Work out the finished part from the listing and answer in its coordinate system (mm). A direction names the side the tool comes from. Give positions to 0.01 mm unless a question says otherwise; leave off trailing zeros. Loops run counter-clockwise (first coordinate to the right, second up) from the corner with the lowest first, then second, coordinate; pieces in that order, holes last. Notation, with made-up numbers: (8, -21) - (58, -21) arc R16 cw to (58, -4) - close; hole circle Ø10 at (62, 6). An arc over 180 degrees is marked (long way). One line per question, with ' | ' between items. Start each with the question number.
1. Each of these flat-tipped pins is pushed along its axis until it touches: pin 1 (1 mm diameter, centred on y = 274, z = 6.5, fed in from -X); pin 2 (1 mm diameter, centred on y = 146, z = 16.5, fed in from -X); pin 3 (3 mm diameter, centred on x = -100.5, z = 47.5, fed in from +Y). Where does it stop, or does it pass through?
2. Which of the six approach directions +Z, -Z, +X, -X, +Y, -Y give full straight-line access (tool end or side, diameter ignored) to faces 1 (the face through (-55, 8, 78.536)), 2 (the face through (-128.253, 304.011, 9.435))?
3. Section D-D (x = -122) is taken. Determine the outline of the cut face in (y, z), plus the area to 3 significant figures.
4. Section C-C (y = 94) is taken. Determine the outline of the cut face in (x, z).
5. Section A-A (z = 29.5) is taken. Determine the outline of the cut face in (x, y).
6. Section B-B (x = -60.5) is taken. Determine the outline of the cut face in (y, z), plus the area to 3 significant figures.
7. Find the intervals of material crossed by line 1 (Z direction, x = 52.85, y = 8); line 2 (Y direction, x = 21, z = 52); line 3 (Z direction, x = -121, y = 312), in increasing order.
Autodesk Inventor part; units mm, degrees
ref_plane "YZ Plane" through (0, 0, 0) normal (1, 0, 0) x (0, 1, 0)
ref_plane "XZ Plane" through (0, 0, 0) normal (0, 1, 0) x (-1, 0, 0)
ref_plane "XY Plane" through (0, 0, 0) normal (0, 0, 1) x (1, 0, 0)
sketch "Sketch1" plane through (0, 0, 0) normal (0, 1, 0) x (-1, 0, 0)
  line L0 (159.7591, 78.536) -> (-52.9659, 78.536)
  line L1 (-52.9659, 78.536) -> (-52.9659, -60.184)
  line L2 (-52.9659, -60.184) -> (159.7591, -60.184)
  line L3 (159.7591, -60.184) -> (159.7591, 78.536)
  point P0 (0, 0)
  dimension "d0" = 138.72
  dimension "d1" = 212.725
extrude "Extrusion1" add sketch "Sketch1" along normal blind 16
sketch "Sketch2" plane through (0, 16, 0) normal (0, 1, 0) x (1, 0, 0)
  line L0 (-159.7591, -78.536) -> (52.9659, -78.536)
  line L1 (52.9659, -78.536) -> (52.9659, 60.184)
  line L2 (52.9659, 60.184) -> (-159.7591, 60.184)
  line L3 (-159.7591, 60.184) -> (-159.7591, -78.536)
  line L4 (-159.7591, 60.184) -> (-159.7591, -78.536)
  line L5 (-159.7591, -9.176) -> (52.9659, -9.176)
  line L6 (52.9659, -78.536) -> (52.9659, 60.184)
  circle A0 centre (-122.3691, -9.176) radius 5.89
  line L7 (-122.3691, -9.176) -> (-128.2591, -9.176)
  point P0 (0, 0)
  dimension "d4" = 11.78
  dimension "d5" = 31.5
extrude "Extrusion2" add sketch "Sketch2" along normal blind 584.2 contours A0 L5 | L5 A0
sketch "Sketch3" plane through (52.9659, 0, 78.536) normal (1, 0, 0) x (0, 0, -1)
  line L0 (0, 0) -> (138.72, 0)
  line L1 (138.72, 0) -> (138.72, 16)
  line L2 (0, 16) -> (138.72, 16)
  line L3 (0, 0) -> (0, 16)
  line L4 (0, 8) -> (138.72, 8)
  circle A0 centre (69.36, 8) radius 3.5
  point P0 (78.536, 0)
  dimension "d8" = 7
extrude "Extrusion3" cut sketch "Sketch3" against normal blind 0.25 contours A0 L4 | L4 A0
properties part number "teststand"
Conclusion:
1) pin 1: x = -127.84 | pin 2: through | pin 3: y = 16
2) face 1: +Z, +X, -X, +Y, -Y | face 2: +Y
3) outline: (0, -60.18) - (16, -60.18) - (16, 3.3) - (600.2, 3.3) - (600.2, 15.05) - (16, 15.05) - (16, 78.54) - (0, 78.54) - close | area: 9,090 mm²
4) outline: circle Ø11.78 at (-122.37, 9.18)
5) outline: (-159.76, 0) - (52.97, 0) - (52.97, 16) - (-159.76, 16) - close
6) outline: (0, -60.18) - (16, -60.18) - (16, 78.54) - (0, 78.54) - close | area: 2,220 mm²
7) line 1: -60.18 to 5.68, 12.68 to 78.54 | line 2: 0 to 16 | line 3: 3.45 to 14.9
